Geometry: final body of the model. Coordinates: model frame, mm. Face numbers are marked on the shaded views. Coordinates: 2 decimals unless noted, no trailing zeros. Write each loop counter-clockwise with the first axis right and the second up, starting at its lowest first coordinate (ties: lowest second). Pieces come first, ordered by that corner, then holes. Notation, with made-up numbers: (36.25, 11) -> (72.25, 11) arc R20 cw to (72.25, 41) -> close; hole circle Ø3 at (59, 43.5). An arc over 180 degrees is marked (long way). One line per item, written item: value. Start each with the question number.
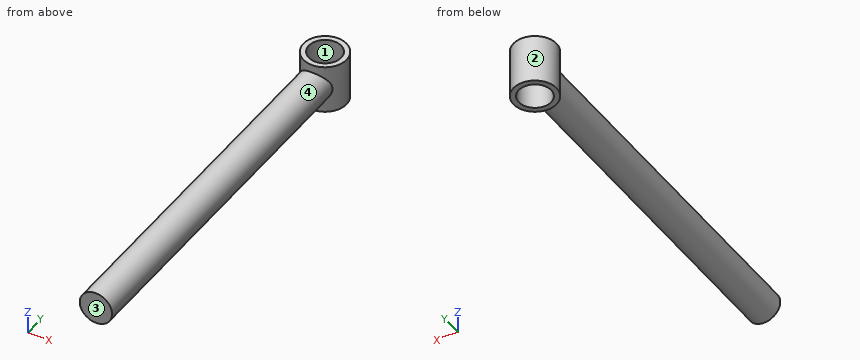
Solid Edge part; units mm, degrees
sketch "Sketch1" plane through (0, 0, 0) normal (0, -1, 0) x (1, 0, 0)
  circle A0 centre (0, 0) radius 30
extrude "ExtrudedProtrusion_1" add sketch "Sketch1" against normal blind 700
sketch "Sketch2" plane through (0, 0, 0) normal (0, 0, 1) x (1, 0, 0)
  circle A0 centre (0, 700) radius 40
extrude "Protrusion1" add sketch "Sketch2" along normal mid plane 90
sketch "Sketch3" plane through (0, 528, 45) normal (0, 0, 1) x (1, 0, 0)
  circle A0 centre (0, 172) radius 30
extrude "Cutout1" cut sketch "Sketch3" against normal through all
Q1. Cut plane B-B on x = 0. Output: boundary loops of the cut face in (y, z).
Q2. Line query: L1, parallel to Y at x = 0, z = 5.5; L2, parallel to Y at x = 0.5, z = -34; L3, parallel to Z at x = 2, y = 412. Output: solid intervals per line, ascending. Write a range as from..to.
Q3. Draft query along Y for the marked faces 1, 2, 3 and 4. Return one class per face: pulls with the +Y half, pulls with the -Y half, needs draft (parallel to the pull), parting line crosses it, or undercut.
Q4. Cut plane A-A on y = 700. Output: boundary loops of the cut face in (x, z), and give its area (3 significant figures).
Q5. First-contact query: P1, Ø4, axis at x = -25, y = 313, coming from the -Z side; P2, Ø1.5, axis at x = -0.5, z = -17.5, coming from the +Y side; P3, Ø6, axis at x = -3.5, y = 154.5, coming from the -Z side. Flat tips, straight axial feed; report the tip coordinate or a pass-through.
Q6. Cut plane C-C on z = 0. Output: boundary loops of the cut face in (x, y), and give its area (3 significant figures).
Q7. Cut plane D-D on y = 338. Output: boundary loops of the cut face in (x, z), and give its area (3 significant figures).
Solution:
1. outline: (0, -30) -> (660, -30) -> (660, -45) -> (670, -45) -> (670, 45) -> (660, 45) -> (660, 30) -> (0, 30) -> close; (730, -45) -> (740, -45) -> (740, 45) -> (730, 45) -> close
2. L1: 0..670, 730..740
2. L2: 660..670, 730..740
2. L3: -29.93..29.93
3. face 1: undercut
3. face 2: parting line crosses it
3. face 3: pulls with the -Y half
3. face 4: needs draft
4. outline: (-40, -45) -> (-30, -45) -> (-30, 45) -> (-40, 45) -> close; (30, -45) -> (40, -45) -> (40, 45) -> (30, 45) -> close
4. area: 1,800 mm²
5. P1: z = -19.26
5. P2: y = 740
5. P3: z = -30
6. outline: (-30, 0) -> (30, 0) -> (30, 673.54) arc R40 ccw (long way) to (-30, 673.54) -> close; hole circle Ø60 at (0, 700)
6. area: 42,000 mm²
7. outline: circle Ø60 at (0, 0)
7. area: 2,830 mm²
